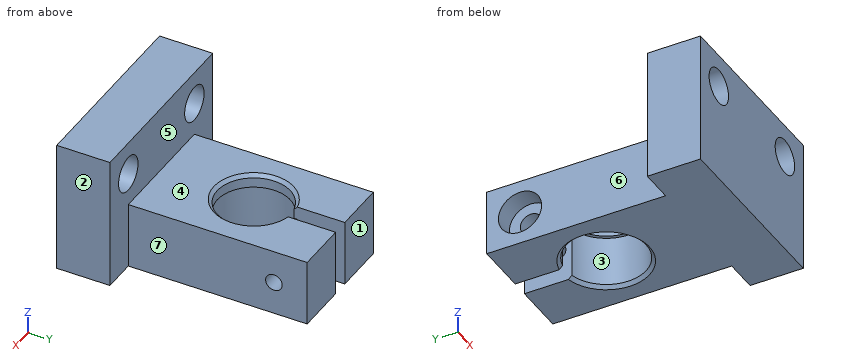
```python
from build123d import *

# Parameters (mm, degrees)
SKETCH1_W                      = 18
SKETCH1_H                      = 34.9
SKETCH1_R                      = 6
BOSS_EXTRUDE1_DEPTH            = 10
BOSS_EXTRUDE2_START            = 2
SKETCH2_R                      = 6
SKETCH2_R_2                    = 5.5
BOSS_EXTRUDE2_DEPTH            = 2
SKETCH3_W                      = 2.5
SKETCH3_H                      = 7.643928679
CUT_EXTRUDE1_DEPTH             = 26.702334524
CBORE_FOR_M3_SHCS1_D           = 3.2
CBORE_FOR_M3_SHCS1_DEPTH       = 7.75
CBORE_FOR_M3_SHCS1_CBORE_D     = 6.5
CBORE_FOR_M3_SHCS1_CBORE_DEPTH = 3
TAP_DRILL_FOR_M3X0_5_TAP1_D    = 2.5
CHAMFER1_SIZE                  = 0.5
SKETCH11_W                     = 10
SKETCH11_H                     = 8
BOSS_EXTRUDE4_DEPTH            = 5
SKETCH8_W                      = 28
SKETCH8_H                      = 10
BOSS_EXTRUDE3_DEPTH            = 8
M5_CLEARANCE_HOLE1_D           = 5.3


with BuildPart() as part:
    # Sketch1 → Boss-Extrude1 (new body)
    with BuildSketch(Plane.XY):
        with Locations((0, -4.45)):
            Rectangle(SKETCH1_W, SKETCH1_H)
        Circle(SKETCH1_R, mode=Mode.SUBTRACT)
    extrude(amount=BOSS_EXTRUDE1_DEPTH)

    # Sketch2 → Boss-Extrude2 (add)
    with BuildSketch(Plane(origin=(0, 0, 10), x_dir=(-1, 0, 0), z_dir=(0, 0, -1)).offset(BOSS_EXTRUDE2_START)):
        Circle(SKETCH2_R)
        Circle(SKETCH2_R_2, mode=Mode.SUBTRACT)
    extrude(amount=-BOSS_EXTRUDE2_DEPTH)

    # Sketch3 → Cut-Extrude1 (cut, through all)
    with BuildSketch(Plane.XY.offset(10)):
        with Locations((0, 9.178035661)):
            Rectangle(SKETCH3_W, SKETCH3_H)
    extrude(amount=-CUT_EXTRUDE1_DEPTH, mode=Mode.SUBTRACT)

    # CBORE for M3 SHCS1
    with Locations(Plane(origin=(9, 0, 0), x_dir=(0, 0, -1), z_dir=(1, 0, 0))):
        with Locations((-5, 8)):
            CounterBoreHole(CBORE_FOR_M3_SHCS1_D / 2, CBORE_FOR_M3_SHCS1_CBORE_D / 2, CBORE_FOR_M3_SHCS1_CBORE_DEPTH, depth=CBORE_FOR_M3_SHCS1_DEPTH)

    # Tap Drill for M3x0.5 Tap1 (through all)
    with Locations(Plane.ZY.offset(9)):
        with Locations((5, 8)):
            Hole(TAP_DRILL_FOR_M3X0_5_TAP1_D / 2)

    # Chamfer1
    chamfer1_edges = [part.edges().sort_by_distance(p)[0] for p in [
        (0, -5.5, 10),
        (0, -6, 0),
    ]]
    chamfer(chamfer1_edges, length=CHAMFER1_SIZE)

    # Sketch11 → Boss-Extrude4 (add)
    with BuildSketch(Plane.ZY.offset(9)):
        with Locations((5, -17.9)):
            Rectangle(SKETCH11_W, SKETCH11_H)
    boss_extrude4 = extrude(amount=BOSS_EXTRUDE4_DEPTH)

    # Mirror1: Boss-Extrude4 across plane
    add(boss_extrude4.mirror(Plane(origin=(0, 0, 0), x_dir=(0, 0, 1), z_dir=(1, 0, 0))))

    # Sketch8 → Boss-Extrude3 (add)
    with BuildSketch(Plane.XZ.offset(21.9)):
        with Locations((0, 15)):
            Rectangle(SKETCH8_W, SKETCH8_H)
    extrude(amount=-BOSS_EXTRUDE3_DEPTH)

    # M5 Clearance Hole1 (through all)
    with Locations(Plane(origin=(0, -13.9, 0), x_dir=(1, 0, 0), z_dir=(0, 1, 0))):
        with Locations((-9, -15), (9, -15)):
            Hole(M5_CLEARANCE_HOLE1_D / 2)


with BuildPart() as body_2:
    # Mirror2: mirrored copy
    add(part.part.mirror(Plane.ZY.offset(-14)))


solid = body_2.part
```
Check sheet for the modelled part. Datum: model origin and axes. Units: mm. Face numbers are marked on the shaded views. A direction names the side the tool comes from. Give positions to 0.01 mm unless a question says otherwise; leave off trailing zeros. Write each loop counter-clockwise with the first axis right and the second up, starting at its lowest first coordinate (ties: lowest second). Pieces come first, ordered by that corner, then holes. Notation, with made-up numbers: (-19, 68) - (-12, 68) arc R25 cw to (-12, 91) - close; hole circle Ø7 at (-5, 83.25). An arc over 180 degrees is marked (long way). Answer as a JSON object with one key per item and string values. Group by question number.
1) Access from +Z, -Z, +X, -X, +Y, -Y to the whole of each face (thin tool, end or side, straight path). Record for the marked faces 4, 5, 6 and 7.
2) Thickness scan on probe 1 along X at (y, z) = (-18.5, 15); probe 2 along X at (y, z) = (8, 2.75); probe 3 along Z at (x, y) = (37, -18). Record the ranges inside material, lowest first. Write a range as from..to.
3) Sectioned sample at A-A (z = 15). Record the cut outline in (x, y).
4) Sectioned sample at B-B (x = 19.5). Record the cut outline in (y, z).
5) Release check for a two-part mould opening along X. For the marked faces 1, 2 and 3 record: pulls with the +X half, pulls with the -X half, needs draft (parallel to the pull), parting line crosses it, or undercut.
6) Depth check by flat-ended pin: P1, Ø5, axis at y = 9, z = 4, coming from the -X side; P2, Ø15.5, axis at x = 28, y = 0, coming from the +Z side; P3, Ø5, axis at y = 8, z = 5, coming from the -X side; P4, Ø2, axis at x = 24.5, y = -16.5, coming from the -Z side. Enter the tip coordinate at first touch or a pass-through.
7) Sectioned sample at C-C (y = 7.5). Record the cut outline in (x, z).
8) Sectioned sample at D-D (x = 28). Record the cut outline in (y, z).
Geometry results:
{
 "1": {"face 4": "+Z, +X, -X, +Y", "face 5": "+Z, +Y", "face 6": "+Z, -Z, -X, +Y", "face 7": "+Z, -Z, +X, +Y"},
 "2": {"probe 1": "x = 14..16.35, 21.65..34.35, 39.65..42", "probe 2": "x = 22..26.75, 29.25..37", "probe 3": "z = 0..12.35, 17.65..20"},
 "3": {"outline": "(14, -21.9) - (16.35, -21.9) - (16.35, -13.9) - (14, -13.9) - close; (21.65, -21.9) - (34.35, -21.9) - (34.35, -13.9) - (21.65, -13.9) - close; (39.65, -21.9) - (42, -21.9) - (42, -13.9) - (39.65, -13.9) - close"},
 "4": {"outline": "(-21.9, 0) - (13, 0) - (13, 10) - (-13.9, 10) - (-13.9, 12.4) - (-21.9, 12.4) - close; (-21.9, 17.6) - (-13.9, 17.6) - (-13.9, 20) - (-21.9, 20) - close; hole circle Ø6.5 at (8, 5)"},
 "5": {"face 1": "needs draft", "face 2": "pulls with the +X half", "face 3": "undercut"},
 "6": {"P1": "stops at x = 19", "P2": "stops at z = 10", "P3": "stops at x = 22", "P4": "stops at z = 0"},
 "7": {"outline": "(19, 0) - (26.75, 0) - (26.75, 3.48) - (22, 3.48) - (22, 1.79) - (19, 1.79) - close; (19, 8.21) - (22, 8.21) - (22, 6.52) - (26.75, 6.52) - (26.75, 10) - (19, 10) - close; (29.25, 0) - (37, 0) - (37, 3.85) - (29.25, 3.85) - close; (29.25, 6.15) - (37, 6.15) - (37, 10) - (29.25, 10) - close"},
 "8": {"outline": "(-21.9, 0) - (-6.5, 0) - (-6, 0.5) - (-6, 8) - (-5.5, 8) - (-5.5, 9.5) - (-6, 10) - (-13.9, 10) - (-13.9, 20) - (-21.9, 20) - close"}
}
